```python
from build123d import *

# Parameters (mm, degrees)
SKETCH1_R               = 2.38125
BOSS_EXTRUDE1_DEPTH     = 1.5875
SKETCH2_W               = 25.4
SKETCH2_H               = 3.175
CUT_EXTRUDE1_DEPTH      = 62.831036149
CUT_EXTRUDE1_DEPTH_BACK = 62.831036149
SKETCH3_W               = 7.9375
SKETCH3_H               = 8.466666666


with BuildPart() as part:
    # Sketch1 → Boss-Extrude1 (new body)
    with BuildSketch(Plane(origin=(0, 0, 0), x_dir=(1, 0, 0), z_dir=(0, 1, 0))):
        with BuildLine():
            Line((-57.15, 12.7), (-57.15, -12.7))
            Line((-57.15, -12.7), (0.697028502, -6.311628258))
            ThreePointArc((0.697028502, -6.311628258), (6.35, 0), (0.697028502, 6.311628258))
            Line((0.697028502, 6.311628258), (-57.15, 12.7))
        make_face()
        with Locations(Location((0, 0, 0), (0, 0, 270))):
            Circle(SKETCH1_R, mode=Mode.SUBTRACT)
        with Locations(Location((-44.45, 6.35, 0), (0, 0, 270))):
            Circle(SKETCH1_R, mode=Mode.SUBTRACT)
        with Locations(Location((-31.75, -4.7625, 0), (0, 0, 270))):
            Circle(SKETCH1_R, mode=Mode.SUBTRACT)
    extrude(amount=BOSS_EXTRUDE1_DEPTH)

    # Sketch2 → Revolve1 (revolve)
    with BuildSketch(Plane.ZY.offset(57.15)):
        with Locations((0, 1.5875)):
            Rectangle(SKETCH2_W, SKETCH2_H)
    revolve(axis=Axis((-57.15, 3.175, -12.7), (0, 0, 1)))

    # Sketch3 → Cut-Extrude1 (cut, two sides: drawn at the far end of the back side and taken through both)
    with BuildSketch(Plane(origin=(0, 1.5875, 0), x_dir=(1, 0, 0), z_dir=(0, 1, 0)).offset(-CUT_EXTRUDE1_DEPTH_BACK)):
        with Locations((-56.35625, 0)):
            Rectangle(SKETCH3_W, SKETCH3_H)
    extrude(amount=CUT_EXTRUDE1_DEPTH + CUT_EXTRUDE1_DEPTH_BACK, mode=Mode.SUBTRACT)


solid = part.part
```
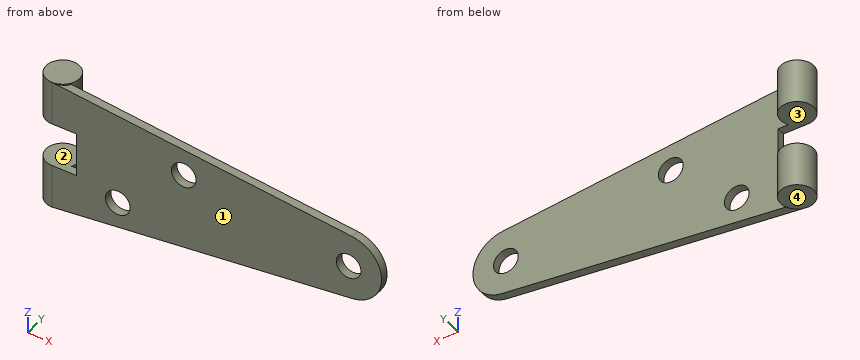
Geometry: final body of the model. Coordinates: model frame, mm. Face numbers are marked on the shaded views. Coordinates: 2 decimals unless noted, no trailing zeros. Order: outer loops, then holes, each group sorted by start corner. A loop starts at its lowest first (then second) coordinate and runs counter-clockwise, first axis right, second up. Notation, with made-up numbers: M 36,11 L 57,11 A27 cw 57,27 Z; hole C 53.5,83.25 d11. An arc over 180 degrees is marked long. Answer in a Markdown table with one row per item. Add a question column.
Q1. Section query D-D on z = -3. Return the cut outline in (x, y).
Q2. Contact query for flat-ended pins moving along their axis: P1, Ø4, axis at x = -31.75, z = 4.76, coming from the +Y side; P2, Ø1.5, axis at x = -38.5, z = -8.5, coming from the +Y side; P3, Ø0.5, axis at y = 0.5, z = 1.5, coming from the -X side; P4, Ø6, axis at x = -50, z = 6.5, coming from the -Y side. Output: stop coordinate, or through.
Q3. Line query: L1, parallel to X at y = 0.4, z = 0; L2, parallel to Z at x = -56.5, y = 3; L3, parallel to Y at x = -23.5, z = 0.5. Output: solid intervals per line, ascending.
Q4. Mould query, pull axis Z, two halves, no side actions, for the marked faces 1, 2, 3 and 4. Classes: released by +Z, released by -Z, zero draft, split by the parting line, or undercut.
Q5. Section query B-B on y = 4. Return the cut outline in (x, z), and give its area (3 significant figures).
Q6. Section query A-A on z = 0. Return the cut outline in (x, y), and give its area (3 significant figures).
Q7. Section query C-C on x = -38.5. Return the cut outline in (y, z).
Completed:
| question | item | result |
|---|---|---|
| 1 | outline | M -52.39,0 L 5.6,0 L 5.6,1.59 L -52.39,1.59 Z |
| 2 | P1 | passes through |
| 2 | P2 | stops at y = 1.59 |
| 2 | P3 | stops at x = -52.39 |
| 2 | P4 | stops at y = 0 |
| 3 | L1 | x = -52.39 to -2.38, 2.38 to 6.35 |
| 3 | L2 | z = -12.7 to -4.23, 4.23 to 12.7 |
| 3 | L3 | y = 0 to 1.59 |
| 4 | face 1 | zero draft |
| 4 | face 2 | undercut |
| 4 | face 3 | undercut |
| 4 | face 4 | released by -Z |
| 5 | outline | M -60.22,-12.7 L -54.08,-12.7 L -54.08,-4.23 L -60.22,-4.23 Z; M -60.22,4.23 L -54.08,4.23 L -54.08,12.7 L -60.22,12.7 Z |
| 5 | area | 104 mm2 |
| 6 | outline | M -52.39,0 L -2.38,0 L -2.38,1.59 L -52.39,1.59 Z; M 2.38,0 L 6.35,0 L 6.35,1.59 L 2.38,1.59 Z |
| 6 | area | 85.7 mm2 |
| 7 | outline | M 0,-10.64 L 1.59,-10.64 L 1.59,10.64 L 0,10.64 Z |
